```python
from build123d import *

# Parameters (mm, degrees)
F1_DEPTH = 50.8
F3_DEPTH = 50.8


with BuildPart() as f1:
    # F0 (on Front) → F1 (new body)
    with BuildSketch(Plane.XZ):
        Polygon((-25.4, 0), (0, 0), (25.4, 0), (25.4, 50.8), (-25.4, 50.8), align=None)
    extrude(amount=F1_DEPTH)

    # F2 (on face) → F3 (cut)
    with BuildSketch(Plane.XZ.offset(50.8)):
        with BuildLine():
            ThreePointArc((0, 50.8), (7.439488, 32.839488), (25.4, 25.4))
            Line((25.4, 25.4), (25.4, 50.8))
            Line((25.4, 50.8), (0, 50.8))
        make_face()
    extrude(amount=-F3_DEPTH, mode=Mode.SUBTRACT)


solid = f1.part
```
Geometry check sheet. Reference: the model listing, model coordinates, mm. Round coordinates to 2 decimals unless told otherwise and drop trailing zeros. Order: outer loops, then holes, each group sorted by start corner. A loop starts at its lowest first (then second) coordinate and runs counter-clockwise, first axis right, second up. Notation, with made-up numbers: (36, 4) - (69, 4) arc R31 cw to (69, 31) - close; hole circle Ø11 at (11.5, 72.5). An arc over 180 degrees is marked (long way). Use a Markdown table: item, result. Add a question column.
(1) Sectioned sample at A-A, the plane y = -37.5. Enter the section's corners in (x, z).
(2) Sectioned sample at B-B, the plane z = 46.5. Enter the section's corners in (x, y), and give its area (3 significant figures).
(3) Sectioned sample at C-C, the plane x = 18. Enter the section's corners in (y, z), and give its area (3 significant figures).
(4) Material ranges on line 1 along X through (y, z) = (-23, 37); line 2 along Z through (x, y) = (17.5, -12); line 3 along Z through (x, y) = (4.5, -18.5), recorded low to high. Write a range as [from, to].
Answers below:
| question | item | result |
|---|---|---|
| 1 | outline | (-25.4, 0) - (25.4, 0) - (25.4, 25.4) arc R25.4 cw to (0, 50.8) - (-25.4, 50.8) - close |
| 2 | outline | (-25.4, -50.8) - (0.37, -50.8) - (0.37, 0) - (-25.4, 0) - close |
| 2 | area | 1,310 mm² |
| 3 | outline | (-50.8, 0) - (0, 0) - (0, 26.5) - (-50.8, 26.5) - close |
| 3 | area | 1,350 mm² |
| 4 | line 1 | [-25.4, 4.08] |
| 4 | line 2 | [0, 26.66] |
| 4 | line 3 | [0, 36.37] |
